```python
from build123d import *

# Parameters (mm, degrees)
SKETCH1_R           = 13
SKETCH1_R_2         = 12
BOSS_EXTRUDE1_DEPTH = 5
REVOLVE1_ANGLE      = 10


with BuildPart() as part:
    # Sketch1 → Boss-Extrude1 (new body)
    with BuildSketch(Plane(origin=(0, 0, 0), x_dir=(1, 0, 0), z_dir=(0, 1, 0))):
        with Locations(Location((0, 0, 0), (0, 0, 270))):
            Circle(SKETCH1_R)
        with Locations(Location((0, 0, 0), (0, 0, 270))):
            Circle(SKETCH1_R_2, mode=Mode.SUBTRACT)
    extrude(amount=BOSS_EXTRUDE1_DEPTH)

    # Sketch2 → Revolve1 (revolve)
    with BuildSketch(Plane.XY):
        Polygon((-13, 5), (-12, 5), (-12, 6.2), (-12, 7.4), (-13.85, 7.4), (-13.85, 6.2), (-13, 6.2), align=None)
        Polygon((12, 6.2), (12, 7.4), (13.85, 7.4), (13.85, 6.2), (13, 6.2), (13, 5), (12, 5), align=None)
    revolve(axis=Axis((0, 0, 0), (0, 1, 0)), revolution_arc=REVOLVE1_ANGLE)


solid = part.part
```
Geometry check sheet. Reference: the model listing, model coordinates, mm. A direction names the side the tool comes from. Round coordinates to 2 decimals unless told otherwise and drop trailing zeros. Write each loop counter-clockwise with the first axis right and the second up, starting at its lowest first coordinate (ties: lowest second). Pieces come first, ordered by that corner, then holes. Notation, with made-up numbers: (83, 34) - (115, 34) arc R35 cw to (115, 67) - close; hole circle Ø1 at (-22.75, -22). An arc over 180 degrees is marked (long way). Write each question's results on one line, items separated by ' | '.
(1) Set-up check for faces 1 (the face through (-12.7, 6.5, 0)), 2 (the face through (12.7, 6.5, 0)), 3 (the face through (-13, 7.4, 1)): record each of +Z, -Z, +X, -X, +Y, -Y from which the full face is reachable in a straight line by a thin tool's end or side.
Computed:
face 1: -Z, -X, +Y | face 2: +Z, +X, +Y | face 3: +Z, -Z, +X, -X, +Y
(2) Sectioned sample at B-B, the plane x = 0. Enter the section's corners in (y, z), plus the area to 3 significant figures.
Computed:
outline: (0, -13) - (5, -13) - (5, -12) - (0, -12) - close; (0, 12) - (5, 12) - (5, 13) - (0, 13) - close | area: 10.0 mm^2
(3) Sectioned sample at A-A, the plane y = 5.5. Enter the section's corners in (x, z).
Computed:
outline: (-13, 0) - (-12, 0) arc R12 cw to (-11.82, 2.08) - (-12.8, 2.26) arc R13 ccw to start; (11.82, -2.08) - (12.8, -2.26) arc R13 ccw to (13, 0) - (12, 0) arc R12 cw to start
(4) Draft check along Z on faces 4 (the face through (12.54, 6.48, -2.21)), 5 (the face through (-12.54, 6.48, 2.21)), 6 (the face through (13, 7.4, -1)). Enter one of: pulls with the +Z half, pulls with the -Z half, needs draft (parallel to the pull), parting line crosses it, or undercut.
Computed:
face 4: pulls with the -Z half | face 5: pulls with the +Z half | face 6: needs draft
(5) Depth check by flat-ended pin: pin 1 Ø8 at (x, z) = (4.5, 2.5) entering from +Y; pin 2 Ø1.5 at (x, y) = (-12.5, 6.5) entering from -Z; pin 3 Ø4 at (x, z) = (-9.5, 4.5) entering from +Y; pin 4 Ø0.5 at (x, z) = (-13.5, 1.5) entering from -Y. Enter the tip coordinate at first touch or a pass-through.
Computed:
pin 1: passes through | pin 2: stops at z = 0 | pin 3: stops at y = 5 | pin 4: stops at y = 6.2
(6) Thickness scan on probe 1 along Z at (x, y) = (0, 3.5); probe 2 along Y at (x, z) = (-8.75, -9.5). Record the ranges inside material, lowest first. Write a range as from..to.
Computed:
probe 1: z = -13..-12, 12..13 | probe 2: y = 0..5
(7) Sectioned sample at D-D, the plane y = 2.75. Enter the section's corners in (x, z).
Computed:
outline: circle Ø26 at (0, 0); hole circle Ø24 at (0, 0)
(8) Sectioned sample at C-C, the plane z = 0.5. Enter the section's corners in (x, y).
Computed:
outline: (-13.84, 6.2) - (-12.99, 6.2) - (-12.99, 0) - (-11.99, 0) - (-11.99, 7.4) - (-13.84, 7.4) - close; (11.99, 0) - (12.99, 0) - (12.99, 5) - (11.99, 5) - close
